```python
from build123d import *

# Parameters (mm, degrees)
F0_R     = 38.1
F0_R_2   = 34.063477528
F1_DEPTH = 101.6
F2_R     = 35.1450557453
F3_DEPTH = 95.25
F4_R     = 10.16
F5_R     = 2.6133627802
F6_DEPTH = 101.601


with BuildPart() as f1:
    # F0 (on Front) → F1 (new body)
    with BuildSketch(Plane.XZ):
        Circle(F0_R)
        Circle(F0_R_2, mode=Mode.SUBTRACT)
        Circle(F0_R_2)
    extrude(amount=F1_DEPTH)

    # F2 (on face) → F3 (cut)
    with BuildSketch(Plane.XZ.offset(101.6)):
        Circle(F2_R)
    extrude(amount=-F3_DEPTH, mode=Mode.SUBTRACT)

    # F4
    f4_edges = [f1.edges().sort_by_distance(p)[0] for p in [
        (-38.1, 0, 0),
    ]]
    fillet(f4_edges, radius=F4_R)

    # F5 (on Front) → F6 (cut, through all)
    with BuildSketch(Plane.XZ):
        Circle(F5_R)
    extrude(amount=F6_DEPTH, mode=Mode.SUBTRACT)


solid = f1.part
```
Geometry: final body of the model. Coordinates: model frame, mm. A direction names the side the tool comes from. Give positions to 0.01 mm unless a question says otherwise; leave off trailing zeros. Order: outer loops, then holes, each group sorted by start corner. A loop starts at its lowest first (then second) coordinate and runs counter-clockwise, first axis right, second up. Notation, with made-up numbers: M 50,-21.5 L 66,-21.5 A22 ccw 66,-15.5 Z; hole C 36,13.5 d8. An arc over 180 degrees is marked long. Answer as CSV lines item,"result". Start each with the question number.
1) First-contact query: P1, Ø8, axis at x = 15.5, z = 27, coming from the +Y side; P2, Ø5, axis at y = -46, z = 24, coming from the +X side; P3, Ø10, axis at y = -32.5, z = -10.5, coming from the -X side; P4, Ø4, axis at x = 15.5, y = -25.5, coming from the -Z side. Flat tips, straight axial feed; report the tip coordinate or a pass-through.
2) Cut plane C-C (y = -14). Output: boundary loops of the cut face in (x, z).
3) Cut plane B-B (x = 0). Output: boundary loops of the cut face in (y, z), then the cut area to 3 significant figures.
4) Mould query, pull axis X, two halves, no side actions, for faces 1 (the cylindrical face through (-30.235, -55.24, -23.183)), 2 (the flat face through (0, -6.35, -7)), 3 (the flat face through (6, 0, 0)). Classes: +X half, -X half, draft (parallel to the pull), parting line (faces both ways), or undercut.
5) Cut plane A-A (z = 0). Output: boundary loops of the cut face in (x, y).
6) Line query: line 1 (Z direction, x = 0, y = -75); line 2 (Y direction, x = 20, z = 10.5); line 3 (X direction, y = -39.5, z = -26). Output: solid intervals per line, ascending. Write a range as from..to.
7) Set-up query: faces 4 (the flat face through (11, -101.6, -34)), 5 (the cylindrical face through (-7.62, -54.64, -34.31)). Return all of +Z, -Z, +X, -X, +Y, -Y with unobstructed straight access to the full face (end or side cutting, diameter ignored); none if empty.
Findings below:
1,P1,"stops at y = 0"
1,P2,"stops at x = 31.45"
1,P3,"stops at x = -37.7"
1,P4,"stops at z = -35.63"
2,outline,"C 0,0 d76.2; hole C 0,0 d70.29"
3,outline,"M -101.6,-38.1 L -10.16,-38.1 A10.16 ccw 0,-27.94 L 0,-2.61 L -6.35,-2.61 L -6.35,-35.15 L -101.6,-35.15 Z; M -101.6,35.15 L -6.35,35.15 L -6.35,2.61 L 0,2.61 L 0,27.94 A10.16 ccw -10.16,38.1 L -101.6,38.1 Z"
3,area,"969 mm²"
4,face 1,"parting line"
4,face 2,"undercut"
4,face 3,"draft"
5,outline,"M -38.1,-101.6 L -35.15,-101.6 L -35.15,-6.35 L -2.61,-6.35 L -2.61,0 L -27.94,0 A10.16 ccw -38.1,-10.16 Z; M 2.61,-6.35 L 35.15,-6.35 L 35.15,-101.6 L 38.1,-101.6 L 38.1,-10.16 A10.16 ccw 27.94,0 L 2.61,0 Z"
6,line 1,"z = -38.1..-35.15, 35.15..38.1"
6,line 2,"y = -6.35..0"
6,line 3,"x = -27.85..-23.65, 23.65..27.85"
7,face 4,"+Z, -Z, +X, -X, -Y"
7,face 5,"-Y"
